```python
from build123d import *

# Parameters (mm, degrees)
BOSS_EXTRUDE2_DEPTH = 5.64


with BuildPart() as part:
    # Sketch1 → Boss-Extrude2 (new body)
    with BuildSketch(Plane.XY):
        with BuildLine():
            Line((-25, 7), (25, 7))
            ThreePointArc((25, 7), (32, 0), (25, -7))
            Line((25, -7), (-25, -7))
            ThreePointArc((-25, -7), (-32, 0), (-25, 7))
        make_face()
        Polygon((-2.020725942, 3.5), (-4.041451884, 0), (-2.020725942, -3.5), (2.020725942, -3.5), (4.041451884, 0), (2.020725942, 3.5), align=None, mode=Mode.SUBTRACT)
    extrude(amount=BOSS_EXTRUDE2_DEPTH)


solid = part.part
```
Geometry: final body of the model. Coordinates: model frame, mm. A direction names the side the tool comes from. Round coordinates to 2 decimals unless told otherwise and drop trailing zeros. Write each loop counter-clockwise with the first axis right and the second up, starting at its lowest first coordinate (ties: lowest second). Pieces come first, ordered by that corner, then holes. Notation, with made-up numbers: M 17,-14 L 46,-14 A38 ccw 46,25 Z; hole C 14,-20.5 d2. An arc over 180 degrees is marked long. Answer in a Markdown table with one row per item. Add a question column.
(1) Cut plane B-B, the plane y = 5.5. Return the cut outline in (x, z).
(2) Cut plane C-C, the plane x = 27. Return the cut outline in (y, z), then the cut area to 3 significant figures.
(3) Reachability of faces 1 (the face through (0, 7, 3)), 2 (the face through (0, -3.5, 3)) from +Z, -Z, +X, -X, +Y, -Y: full face, straight path, thin tool, end or side. Return the list, or none.
(4) Cut plane A-A, the plane z = 1.4. Return the cut outline in (x, y).
(5) Ray query, L1, parallel to Y at x = 0, z = 0.5; L2, parallel to X at y = -1.75, z = 2.3; L3, parallel to X at y = -0.25, z = 2.4. Return the intervals inside material, ascending.
(6) Draft query along X for faces 3 (the face through (-32, 0, 3)), 4 (the face through (3, -1.8, 2.8)), 5 (the face through (0, -7, 3)), 6 (the face through (-3, 1.8, 2.8)). Return one class per face: pulls with the +X half, pulls with the -X half, needs draft (parallel to the pull), parting line crosses it, or undercut.
Established:
| question | item | result |
|---|---|---|
| 1 | outline | M -29.33,0 L 29.33,0 L 29.33,5.64 L -29.33,5.64 Z |
| 2 | outline | M -6.71,0 L 6.71,0 L 6.71,5.64 L -6.71,5.64 Z |
| 2 | area | 75.7 mm² |
| 3 | face 1 | +Z, -Z, +X, -X, +Y |
| 3 | face 2 | +Z, -Z |
| 4 | outline | M -25,-7 L 25,-7 A7 ccw 25,7 L -25,7 A7 ccw Z; hole M -4.04,0 L -2.02,-3.5 L 2.02,-3.5 L 4.04,0 L 2.02,3.5 L -2.02,3.5 Z |
| 5 | L1 | -7 to -3.5, 3.5 to 7 |
| 5 | L2 | -31.78 to -3.03, 3.03 to 31.78 |
| 5 | L3 | -32 to -3.9, 3.9 to 32 |
| 6 | face 3 | pulls with the -X half |
| 6 | face 4 | undercut |
| 6 | face 5 | needs draft |
| 6 | face 6 | undercut |
